from build123d import *

# Parameters (mm, degrees)
CHAMFER1_SIZE      = 0.5
CHAMFER2_SIZE      = 0.3
CUT_EXTRUDE1_DEPTH = 2.5
CHAMFER3_SIZE      = 0.3


with BuildPart() as part:
    # Sketch1 → Revolve1 (revolve)
    with BuildSketch(Plane.XY):
        Polygon((0, 0), (0, 2.75), (3, 2.75), (3, 1.49), (18, 1.49), (18, 0), align=None)
    revolve(axis=Axis((-88.705490849, 0, 0), (1, 0, 0)))

    # Chamfer1
    chamfer1_edges = [part.edges().sort_by_distance(p)[0] for p in [
        (18, -1.49, 0),
    ]]
    chamfer(chamfer1_edges, length=CHAMFER1_SIZE)

    # Chamfer2
    chamfer2_edges = [part.edges().sort_by_distance(p)[0] for p in [
        (0, -2.75, 0),
    ]]
    chamfer(chamfer2_edges, length=CHAMFER2_SIZE)

    # Sketch3 → Cut-Extrude1 (cut)
    with BuildSketch(Plane(origin=(0, 0, 0), x_dir=(0, 0, -1), z_dir=(1, 0, 0))):
        Polygon((-1.443375673, 0), (-0.721687836, -1.25), (0.721687836, -1.25), (1.443375673, 0), (0.721687836, 1.25), (-0.721687836, 1.25), align=None)
    extrude(amount=CUT_EXTRUDE1_DEPTH, mode=Mode.SUBTRACT)

    # Chamfer3
    chamfer3_edges = [part.edges().sort_by_distance(p)[0] for p in [
        (0, 0.625, 1.082531755),
        (0, -0.625, 1.082531755),
        (0, -1.25, 0),
        (0, -0.625, -1.082531755),
        (0, 0.625, -1.082531755),
        (0, 1.25, 0),
    ]]
    chamfer(chamfer3_edges, length=CHAMFER3_SIZE)


solid = part.part
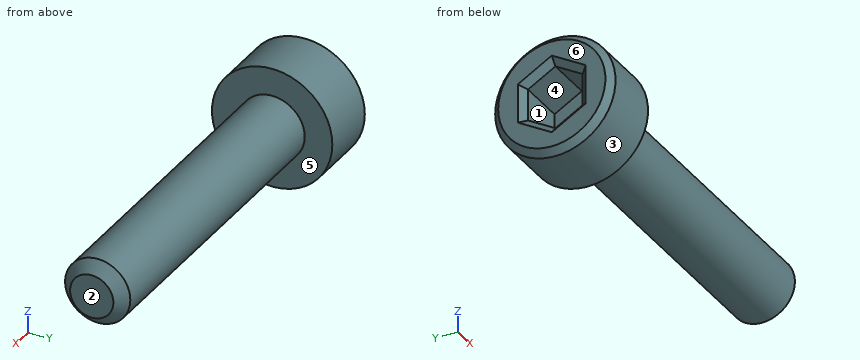
The model under review builds one solid part; all positions refer to its coordinate system, in mm. Face numbers are marked on the shaded views. A direction names the side the tool comes from. Give positions to 0.01 mm unless a question says otherwise; leave off trailing zeros. Loops run counter-clockwise (first coordinate to the right, second up) from the corner with the lowest first, then second, coordinate; pieces in that order, holes last. Notation, with made-up numbers: (-27, 54.25) -> (-14, 54.25) arc R29 ccw to (-14, 78.25) -> close; hole circle Ø2 at (62.5, -5). An arc over 180 degrees is marked (long way). Put each result on its own line as item: value. Start each with the question number.
1. Wall thickness on probe 1 along Z at (x, y) = (10.25, -0.35); probe 2 along Y at (x, z) = (1.75, -1.2); probe 3 along X at (y, z) = (-1, -1.25): over which ranges is each line inside the solid? List them lowest first.
2. For the marked faces 5 and 6, list the 3-axis set-ups (+Z, -Z, +X, -X, +Y, -Y) from which the entire face can be reached by the end or side of a thin tool; tool diameter is ignored.
3. We need section A-A on z = 0. State the section outline as (x, y) points, then the cut area to 3 significant figures.
4. We need section B-B on x = 7.5. State the section outline as (y, z) points.
5. Clearance check with flat-ended pins moving along their axes: P1, Ø0.8, axis at y = 0.5, z = 0, coming from the -X side; P2, Ø3, axis at x = 12, z = 2, coming from the +Y side; P3, Ø1, axis at y = 1.5, z = 1, coming from the +X side. State where each tip first meets the part, or that it passes through.
6. Mouldability with a two-part tool opening along Z and no side actions: class the marked faces 1, 2, 3 and 4 as released by +Z, released by -Z, zero draft, split by the parting line, or undercut.
Determined:
1. probe 1: -1.45 to 1.45
1. probe 2: -2.47 to -0.42, 0.42 to 2.47
1. probe 3: 0 to 3
2. face 5: +X
2. face 6: +Z, -Z, -X, +Y, -Y
3. outline: (0, -2.45) -> (0.3, -2.75) -> (3, -2.75) -> (3, -1.49) -> (17.5, -1.49) -> (18, -0.99) -> (18, 0.99) -> (17.5, 1.49) -> (3, 1.49) -> (3, 2.75) -> (0.3, 2.75) -> (0, 2.45) -> (0, 1.55) -> (0.3, 1.25) -> (2.5, 1.25) -> (2.5, -1.25) -> (0.3, -1.25) -> (0, -1.55) -> close
3. area: 54.5 mm^2
4. outline: circle Ø2.98 at (0, 0)
5. P1: x = 2.5
5. P2: y = 1.4
5. P3: x = 17.69
6. face 1: undercut
6. face 2: zero draft
6. face 3: split by the parting line
6. face 4: undercut
